Autodesk Inventor part; units mm, degrees
ref_plane "YZ Plane" through (0, 0, 0) normal (1, 0, 0) x (0, 1, 0)
ref_plane "XZ Plane" through (0, 0, 0) normal (0, 1, 0) x (-1, 0, 0)
ref_plane "XY Plane" through (0, 0, 0) normal (0, 0, 1) x (1, 0, 0)
sketch "Sketch1" plane through (0, 0, 0) normal (0, 0, 1) x (1, 0, 0)
  line L0 (0, 0) -> (0, 55) construction
  circle A0 centre (0, 47.5) radius 7.5 construction
  circle A1 centre (0, 7.5) radius 7.5 construction
  line L1 (7.5, 47.5) -> (7.5, 7.5)
  line L2 (-7.5, 7.5) -> (-7.5, 47.5)
  arc A2 (7.5, 47.5) -> (-7.5, 47.5) centre (0, 47.5) ccw
  arc A3 (-7.5, 7.5) -> (7.5, 7.5) centre (0, 7.5) ccw
  circle A4 centre (0, 27.5) radius 3.9
  circle A5 centre (0, 47.5) radius 1.75
  circle A6 centre (0, 7.5) radius 1.75
  dimension "d1" = 15
  dimension "d2" = 15
  dimension "d3" = 7.8
  dimension "d4" = 3.5
  dimension "d5" = 3.5
  dimension "d21" = 40
extrude "Extrusion1" add sketch "Sketch1" along normal blind 3
sketch "Sketch3" plane through (0, 0, 0) normal (0, 0, -1) x (-1, 0, 0)
  circle A0 centre (0, 47.5) radius 1.75
  circle A1 centre (0, 7.5) radius 1.75
  point P0 (0, 0)
extrude "Extrusion2" add sketch "Sketch3" against normal blind 9
sketch "Sketch4" plane through (0, 47.5, 9) normal (0, 0, 1) x (1, 0, 0)
  circle A0 centre (0, 0) radius 1.75
  circle A1 centre (0, -40) radius 1.75
  circle A2 centre (0, 0) radius 1
  circle A3 centre (0, -40) radius 1
  point P0 (0, -47.5)
  dimension "d10" = 2
  dimension "d11" = 2
extrude "Extrusion3" cut sketch "Sketch4" against normal through all contours A2 | A3
sketch "Sketch5" plane through (0, 0, 3) normal (0, 0, 1) x (1, 0, 0)
  arc A0 (7.5, 47.5) -> (-7.5, 47.5) centre (0, 47.5) ccw
  arc A1 (-7.5, 7.5) -> (7.5, 7.5) centre (0, 7.5) ccw
  circle A2 centre (0, 47.5) radius 1
  circle A3 centre (0, 47.5) radius 11 construction
  circle A4 centre (0, 7.5) radius 11 construction
  line L0 (7.5, 7.5) -> (7.5, 47.5)
  line L1 (7.5, 39.4533) -> (7.5, 15.5467)
  line L2 (-7.5, 47.5) -> (-7.5, 7.5)
  line L3 (-7.5, 39.4533) -> (-7.5, 15.5467)
  arc A5 (-7.5, 39.4533) -> (7.5, 39.4533) centre (0, 47.5) ccw
  arc A6 (7.5, 15.5467) -> (-7.5, 15.5467) centre (0, 7.5) ccw
  circle A7 centre (0, 27.5) radius 3.9
  point P0 (0, 0)
  dimension "d14" = 22
  dimension "d15" = 22
extrude "Extrusion4" add sketch "Sketch5" along normal blind 6 contours L0 A6 L2 A5
sketch "Sketch6" plane through (0, 0, 0) normal (1, 0, 0) x (0, 1, 0)
  line L0 (7.5, 0) -> (47.5, 0)
  line L1 (7.5, 0) -> (7.5, 3)
  line L2 (15.5467, 3) -> (7.5, 3)
  line L3 (15.5467, 3) -> (15.5467, 9)
  line L4 (39.4533, 9) -> (15.5467, 9)
  line L5 (39.4533, 3) -> (39.4533, 9)
  line L6 (47.5, 0) -> (47.5, 3)
  circle A0 centre (27.5, 6) radius 1.5
  line L7 (47.5, 3) -> (39.4533, 3)
  point P0 (0, 0)
  point P1 (27.5, 9)
  point P2 (39.4533, 6)
  dimension "d18" = 3
extrude "Extrusion5" cut sketch "Sketch6" against normal through all contours A0
equation "\"d5\" = d4"
equation "\"d15\" = d14"
properties part number "WaveGenerator" material "ABS Plastic"
The model under review builds one solid part; all positions refer to its coordinate system, in mm. A direction names the side the tool comes from. Give positions to 0.01 mm unless a question says otherwise; leave off trailing zeros. Order: outer loops, then holes, each group sorted by start corner. A loop starts at its lowest first (then second) coordinate and runs counter-clockwise, first axis right, second up. Notation, with made-up numbers: (31, 40.25) -> (38, 40.25) arc R23 cw to (38, 55.25) -> close; hole circle Ø4 at (-26, 51.25). An arc over 180 degrees is marked (long way). Write item = value, one per line. Start each with the question number.
(1) Take a section at A-A (z = 3.75). Write out the cut boundary in (x, y).
(2) Take a section at D-D (z = 6.75). Write out the cut boundary in (x, y).
(3) For pin 1 Ø1 at (x, z) = (2.5, 1.5) entering from +Y; pin 2 Ø1.5 at (x, z) = (-0.5, 7) entering from -Y, all flat-tipped, find the tip position at first contact; note any pin that passes through.
(4) Draft analysis for pull direction X (two halves, no side actions). For faces 4 (the cylindrical face through (-0.13, 48.49, 4.56)), 5 (the flat face through (5, 28, 0)), 6 (the cylindrical face through (0.1, 36.5, 6)), 7 (the flat face through (7.5, 27, 3)), state which applies: +X half, -X half, draft (parallel to the pull), parting line (faces both ways), or undercut.
(5) Tool access review of faces 1 (the cylindrical face through (-0.13, 8.49, 4.56)), 2 (the cylindrical face through (-6, 26, 6)), 3 (the cylindrical face through (0.38, 5.79, 5.96)): name each direction out of +Z, -Z, +X, -X, +Y, -Y from which nothing blocks a thin tool from reaching the whole face with its end or side.
(6) Take a section at B-B (x = 0). Write out the cut boundary in (y, z).
(7) Take a section at C-C (y = 27.5). Write out the cut boundary in (x, z).
(8) For L1, parallel to Y at x = 0, z = 3.75; L2, parallel to Z at x = -5.65, y = 27.5; L3, parallel to Z at x = 2.25, y = 17, list the stretches that pass through material, from the lowest coordinate up. Write a range as from..to.
Returned:
q1.outline = (-7.5, 15.55) arc R11 cw to (7.5, 15.55) -> (7.5, 39.45) arc R11 cw to (-7.5, 39.45) -> close; circle Ø3.5 at (0, 7.5); circle Ø3.5 at (0, 47.5); hole circle Ø7.8 at (0, 27.5); hole circle Ø2 at (0, 7.5); hole circle Ø2 at (0, 47.5)
q2.outline = (-7.5, 15.55) arc R11 cw to (7.5, 15.55) -> (7.5, 39.45) arc R11 cw to (-7.5, 39.45) -> (-7.5, 28.8) -> (-3.68, 28.8) arc R3.9 cw (long way) to (-3.68, 26.2) -> (-7.5, 26.2) -> close; circle Ø3.5 at (0, 7.5); circle Ø3.5 at (0, 47.5); hole circle Ø2 at (0, 7.5); hole circle Ø2 at (0, 47.5)
q3.pin_1 = 54.73
q3.pin_2 = 5.75
q4.face_4 = undercut
q4.face_5 = draft
q4.face_6 = undercut
q4.face_7 = +X half
q5.face_1 = +Z, -Z
q5.face_2 = -X
q5.face_3 = +Z
q6.outline = (0, 0) -> (6.5, 0) -> (6.5, 9) -> (5.75, 9) -> (5.75, 3) -> (0, 3) -> close; (8.5, 0) -> (23.6, 0) -> (23.6, 9) -> (18.5, 9) -> (18.5, 3) -> (9.25, 3) -> (9.25, 9) -> (8.5, 9) -> close; (31.4, 0) -> (46.5, 0) -> (46.5, 9) -> (45.75, 9) -> (45.75, 3) -> (36.5, 3) -> (36.5, 9) -> (31.4, 9) -> close; (48.5, 0) -> (55, 0) -> (55, 3) -> (49.25, 3) -> (49.25, 9) -> (48.5, 9) -> close
q7.outline = (-7.5, 0) -> (-3.9, 0) -> (-3.9, 4.5) -> (-7.5, 4.5) -> close; (-7.5, 7.5) -> (-3.9, 7.5) -> (-3.9, 9) -> (-7.5, 9) -> close; (3.9, 0) -> (7.5, 0) -> (7.5, 9) -> (3.9, 9) -> close
q8.L1 = 5.75..6.5, 8.5..9.25, 18.5..23.6, 31.4..36.5, 45.75..46.5, 48.5..49.25
q8.L2 = 0..4.5, 7.5..9
q8.L3 = 0..3
